The listing builds one solid part. Answer for the finished solid, in the listing's coordinates (mm). Face numbers are marked on the shaded views. A direction names the side the tool comes from. Round coordinates to 2 decimals unless told otherwise and drop trailing zeros. Order: outer loops, then holes, each group sorted by start corner. A loop starts at its lowest first (then second) coordinate and runs counter-clockwise, first axis right, second up. Notation, with made-up numbers: M 59.5,48.25 L 91.5,48.25 A11 ccw 91.5,58.25 Z; hole C -14.5,28.25 d7. An arc over 180 degrees is marked long. Write item = value, one per line. Start each with the question number.
(1) Each of these flat-tipped pins is pushed along its axis until it touches: pin 1 (3.5 mm diameter, centred on y = 10, z = -7, fed in from +X); pin 2 (2.5 mm diameter, centred on y = 19.5, z = -7, fed in from -X); pin 3 (3.5 mm diameter, centred on y = 19, z = -7.5, fed in from +X); pin 4 (3 mm diameter, centred on x = 25, z = -8.5, fed in from -Y). Where does it stop, or does it pass through?
(2) Which of the six approach directions +Z, -Z, +X, -X, +Y, -Y give full straight-line access (tool end or side, diameter ignored) to the marked faces 4, 5, 6, 7 and 8?
(3) A cutting plane is placed at B-B, the plane y = 18. Determine the outline of the cut face in (x, z), and give its area (3 significant figures).
(4) A cutting plane is placed at C-C, the plane z = -3.75. Determine the outline of the cut face in (x, y).
(5) Straight lines are drawn through the part: probe 1 along X at (y, z) = (10.25, -6); probe 2 along Z at (x, y) = (6, 18.75); probe 3 along Y at (x, z) = (13.5, -1). For each, find the intervals that lie inside material, in ascending order. Write a range as from..to.
(6) For a pull along Z with two mould halves and no side action, classify the marked faces 1, 2 and 3 as released by +Z, released by -Z, zero draft, split by the parting line, or undercut.
(7) A cutting plane is placed at D-D, the plane x = 1. Determine the outline of the cut face in (y, z), and give its area (3 significant figures).
Autodesk Inventor part; units mm, degrees
ref_plane "YZ Plane" through (0, 0, 0) normal (1, 0, 0) x (0, 1, 0)
ref_plane "XZ Plane" through (0, 0, 0) normal (0, 1, 0) x (-1, 0, 0)
ref_plane "XY Plane" through (0, 0, 0) normal (0, 0, 1) x (1, 0, 0)
sketch "スケッチ1" plane through (0, 0, 0) normal (0, 1, 0) x (-1, 0, 0)
  line L0 (0, 0) -> (-23, 0)
  line L1 (-23, 0) -> (-23, -12)
  line L2 (-23, -12) -> (0, -12)
  line L3 (0, -12) -> (0, 0)
  dimension "d0" = 23
  dimension "d1" = 12
extrude "押し出し1" add sketch "スケッチ1" along normal blind 16.5
sketch "スケッチ2" plane through (0, 16.5, 0) normal (0, 1, 0) x (1, 0, 0)
  line L0 (23, 0) -> (23, 12)
  line L1 (23, 12) -> (0, 12)
  line L2 (0, 12) -> (0, 0)
  line L3 (0, 0) -> (23, 0)
  line L4 (-4, 0) -> (27, 0)
  line L5 (27, 0) -> (27, 12)
  line L6 (27, 12) -> (-4, 12)
  line L7 (-4, 12) -> (-4, 0)
  dimension "d4" = 4
  dimension "d5" = 4
extrude "押し出し2" add sketch "スケッチ2" along normal blind 1
sketch "スケッチ3" plane through (0, 17.5, 0) normal (0, 1, 0) x (1, 0, 0)
  line L0 (-4, 0) -> (27, 0)
  line L1 (27, 12) -> (-4, 12)
  line L2 (0, 12) -> (0, 0)
  line L3 (23, 0) -> (23, 12)
extrude "押し出し3" add sketch "スケッチ3" along normal blind 3
sketch "スケッチ4" plane through (0, 20.5, 0) normal (0, 1, 0) x (1, 0, 0)
  line L0 (23, 12) -> (0, 12)
  line L1 (0, 12) -> (0, 0)
  line L2 (0, 0) -> (23, 0)
  circle A0 centre (6, 6) radius 6
extrude "押し出し4" add sketch "スケッチ4" along normal blind 3 contours A0
sketch "スケッチ5" plane through (6, 23.5, -6) normal (0, 1, 0) x (1, 0, 0)
  circle A0 centre (0, 0) radius 6
  point P0 (-6, -6)
hole "穴1" at (6, 23.5, -6) direction (0, -1, 0) diameter 3 end through all
equation "\"d5\" = d4"
properties part number "ServoMotor_8g"
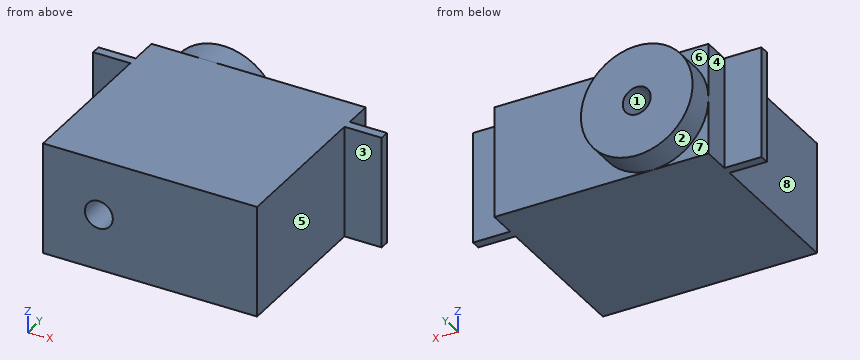
Reported:
q1.pin_1 = 23
q1.pin_2 = 0
q1.pin_3 = 27
q1.pin_4 = 16.5
q2.face_4 = +Z, -Z, -X, +Y
q2.face_5 = +Z, -Z, +X, -Y
q2.face_6 = +Z, -X, +Y
q2.face_7 = -Z, -X, +Y
q2.face_8 = +Z, -Z, -X, -Y
q3.outline = M 0,-12 L 23,-12 L 23,0 L 0,0 Z; hole C 6,-6 d3
q3.area = 269 mm²
q4.outline = M -4,16.5 L 0,16.5 L 0,0 L 23,0 L 23,16.5 L 27,16.5 L 27,17.5 L 23,17.5 L 23,20.5 L 11.56,20.5 L 11.56,23.5 L 0.44,23.5 L 0.44,20.5 L 0,20.5 L 0,17.5 L -4,17.5 Z
q5.probe_1 = 0..4.5, 7.5..23
q5.probe_2 = -12..-7.5, -4.5..0
q5.probe_3 = 0..20.5
q6.face_1 = undercut
q6.face_2 = split by the parting line
q6.face_3 = zero draft
q7.outline = M 0,-12 L 20.5,-12 L 20.5,-9.32 L 23.5,-9.32 L 23.5,-2.68 L 20.5,-2.68 L 20.5,0 L 0,0 Z
q7.area = 266 mm²
